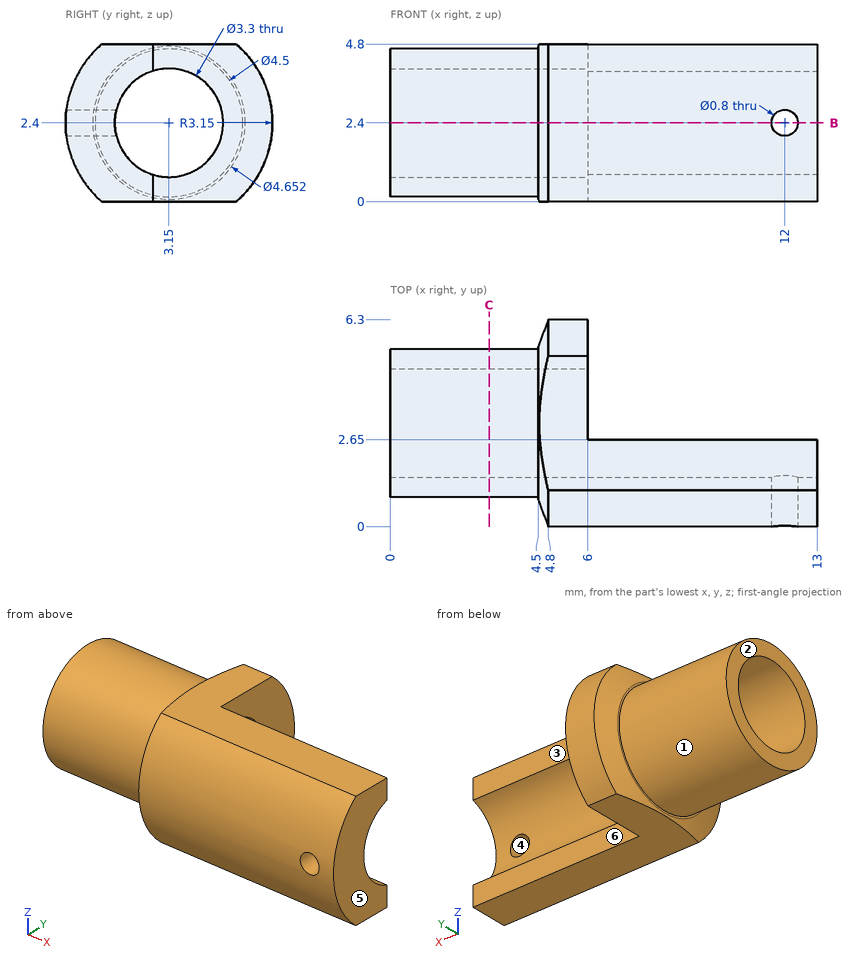
Check sheet for the drawn part. Datum: minimum x, y, z corner. Units: mm. A direction names the side the tool comes from. Coordinates: 2 decimals unless noted, no trailing zeros. Loops run counter-clockwise (first coordinate to the right, second up) from the corner with the lowest first, then second, coordinate; pieces in that order, holes last. Notation, with made-up numbers: (83, 87.25) -> (118, 87.25) arc R12 cw to (118, 105.25) -> close; hole circle Ø11 at (-28, -24.5). An arc over 180 degrees is marked (long way). Answer as CSV lines item,"result".
1) Cross-section at B-B, the plane z = 2.4. Count the separate pieces of the cut face and the enclosed holes in it.
Found:
separate pieces,"3"
enclosed holes,"0"
2) Thickness scan on L1, parallel to Z at x = 5.25, y = 3.15; L2, parallel to Z at x = 2.75, y = 3.15; L3, parallel to Y at x = 10, z = 2.4. Record the ranges inside material, lowest first. Write a range as from..to.
Found:
L1,"z = 0..0.75, 4.05..4.8"
L2,"z = 0.15..0.75, 4.05..4.65"
L3,"y = 0..1.5"
3) Release check for a two-part mould opening along X. For the marked faces 4, 5 and 6 record: +X half, -X half, draft (parallel to the pull), parting line (faces both ways), or undercut.
Found:
face 4,"undercut"
face 5,"+X half"
face 6,"draft"
4) Depth check by flat-ended pin: pin 1 (2 mm diameter, centred on x = 9, z = 0.5, fed in from -Y); pin 2 (1 mm diameter, centred on x = 5, y = 5.5, fed in from -Z); pin 3 (0.9 mm diameter, centred on x = 10, z = 4.5, fed in from +Y); pin 4 (2 mm diameter, centred on x = 2.5, z = 4, fed in from +Y). Enter the tip coordinate at first touch or a pass-through.
Found:
pin 1,"stops at y = 0.13"
pin 2,"stops at z = 0"
pin 3,"stops at y = 2.65"
pin 4,"stops at y = 5.32"
5) Cross-section at C-C, the plane x = 3. Record the cut outline in (y, z).
Found:
outline,"circle Ø4.5 at (3.15, 2.4); hole circle Ø3.3 at (3.15, 2.4)"
6) Tool access check on the marked faces 1, 2 and 3. Record the directions out of +Z, -Z, +X, -X, +Y, -Y that give a thin tool (end or side, any length) a straight path to the whole face; none if there is none.
Found:
face 1,"-X"
face 2,"+Z, -Z, -X, +Y, -Y"
face 3,"+Z, -Z, +X, +Y"
